For this review, take the finished solid that the model builds, in its own axes (mm). A direction names the side the tool comes from. Round coordinates to 2 decimals unless told otherwise and drop trailing zeros. Loops run counter-clockwise (first coordinate to the right, second up) from the corner with the lowest first, then second, coordinate; pieces in that order, holes last.
1. To check wall thickness, follow line 1 along X through (y, z) = (1.5, -3); line 2 along X through (y, z) = (-0.25, 1.75); line 3 along Y through (x, z) = (3, 2.25). State the ranges of each line that lie inside material, in increasing order.
2. Clearance check with flat-ended pins moving along their axes: pin 1 Ø1.5 at (x, z) = (-1.5, -1.5) entering from -Y; pin 2 Ø0.5 at (y, z) = (1, 1.5) entering from -X; pin 3 Ø0.7 at (x, y) = (-4, 0.5) entering from -Z. State where each tip first meets the part, or that it passes through.
3. Consider section A-A on x = 8. State the section outline as (y, z) points, then the cut area to 3 significant figures.
4. Draft analysis for pull direction Z (two halves, no side actions). For faces 4 (the flat face through (-3, 0, 2)), 5 (the flat face through (-5, 2, -2)), 6 (the cylindrical face through (6.11, -0.54, -2.44)), state which applies: released by +Z, released by -Z, zero draft, split by the parting line, or undercut.
5. Tool access review of faces 1 (the cylindrical face through (-2.218, 2.285, 3.584)), 2 (the flat face through (-3.43, 1.74, 0.99)), 3 (the flat face through (0, 0, -3)): name each direction out of +Z, -Z, +X, -X, +Y, -Y from which nothing blocks a thin tool from reaching the whole face with its end or side.
Autodesk Inventor part; units mm, degrees
ref_plane "IP1_XY" through (0, 0, 0) normal (1, 0, 0) x (0, 0, -1)
ref_plane "IP1_YZ" through (0, 0, 0) normal (0, 0, -1) x (0, 1, 0)
ref_plane "IP1_ZX" through (0, 0, 0) normal (0, 1, 0) x (1, 0, 0)
sketch "Skizze_2" plane through (0, 0, 0) normal (0, 0, 1) x (1, 0, 0)
  line L0 (12, 0) -> (-8, 0)
  line L1 (-0.7453, 0) -> (-1.9, 2)
  line L2 (-1.9, 2) -> (-5, 2)
  line L3 (-5, 2) -> (-5, 3.75)
  arc A0 (-4.5, 4.25) -> (-5, 3.75) centre (-4.5, 3.75) ccw
  line L4 (-4.5, 4.25) -> (0, 4.25)
  line L5 (0, 4.25) -> (0, 2.7114)
  line L6 (0, 2.7114) -> (0.5637, 2.5)
  line L7 (0.5637, 2.5) -> (11.5095, 2.5)
  line L8 (11.5095, 2.5) -> (12, 2.0095)
  line L9 (12, 2.0095) -> (12, 0)
  line L10 (12, 0) -> (-0.7453, 0)
revolve "Revolution1" add sketch "Skizze_2" angle 360 about axis through (12, 0, 0) along (1, 0, 0)
thread "Thread1"
sketch "Skizze_1" plane through (-1.9, 0, 0) normal (1, 0, 0) x (0, 0, -1)
  line L0 (-2, 1.1547) -> (-2, -1.1547)
  line L1 (-2, -1.1547) -> (0, -2.3094)
  line L2 (0, -2.3094) -> (2, -1.1547)
  line L3 (2, -1.1547) -> (2, 1.1547)
  line L4 (2, 1.1547) -> (0, 2.3094)
  line L5 (0, 2.3094) -> (-2, 1.1547)
extrude "Extrusion1" cut sketch "Skizze_1" against normal blind 5
ref_plane "IP1_XY" through (0, 0, 0) normal (1, 0, 0) x (0, 0, -1)
ref_plane "IP1_YZ" through (0, 0, 0) normal (0, 0, -1) x (0, 1, 0)
ref_plane "IP1_ZX" through (0, 0, 0) normal (0, 1, 0) x (1, 0, 0)
ref_plane "IP2_XY" through (-5, 0, 0) normal (1, 0, 0) x (0, 0, -1)
ref_plane "IP2_YZ" through (-5, 0, 0) normal (0, 0, -1) x (0, 1, 0)
ref_plane "IP2_ZX" through (-5, 0, 0) normal (0, 1, 0) x (1, 0, 0)
ref_plane "IP3_XY" through (12, 0, 0) normal (1, 0, 0) x (0, 0, -1)
ref_plane "IP3_YZ" through (12, 0, 0) normal (0, 0, -1) x (0, 1, 0)
ref_plane "IP3_ZX" through (12, 0, 0) normal (0, 1, 0) x (1, 0, 0)
ref_plane "IP4_XY" through (0, 0, 0) normal (1, 0, 0) x (0, 0, -1)
ref_plane "IP4_YZ" through (0, 0, 0) normal (0, 0, -1) x (0, 1, 0)
ref_plane "IP4_ZX" through (0, 0, 0) normal (0, 1, 0) x (1, 0, 0)
properties part number "Zylinderschraube ISO 4762 - screw - M5x12-screw"
Resolved:
1. line 1: x = -5 to 0
1. line 2: x = -1.77 to 12
1. line 3: y = -1.09 to 1.09
2. pin 1: stops at y = -4.18
2. pin 2: stops at x = -1.9
2. pin 3: stops at z = -4.25
3. outline: circle Ø5 at (0, 0)
3. area: 19.6 mm2
4. face 4: undercut
4. face 5: zero draft
4. face 6: split by the parting line
5. face 1: +X, -X
5. face 2: -X
5. face 3: +X
